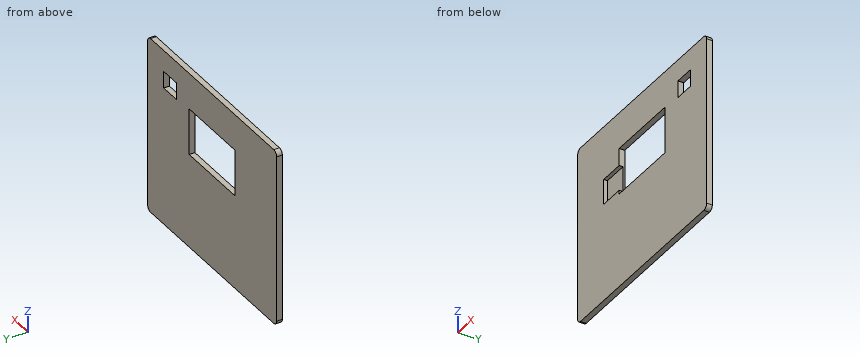
```python
from build123d import *

# Parameters (mm, degrees)
SKETCH_1_W               = 670
SKETCH_1_H               = 560
EXTRUDE_1_DEPTH          = 18
CUT_EXTRUDE_1_DEPTH      = 653.80088848
CUT_EXTRUDE_1_DEPTH_BACK = 653.80088848
SKETCH_2_W               = 65.5
SKETCH_2_H               = 53.5
CUT_EXTRUDE_2_DEPTH      = 653.80088848
CUT_EXTRUDE_2_DEPTH_BACK = 653.80088848
SKETCH_3_W               = 228
SKETCH_3_H               = 136
CUT_EXTRUDE_3_REACH      = 654.801
SKETCH_4_W               = 239
SKETCH_4_H               = 147
FILLET_1_R               = 15
SKETCH_8_W               = 80.472707968
SKETCH_8_H               = 80
CUT_EXTRUDE_4_DEPTH      = 12


with BuildPart() as part:
    # 草图1 → 凸台-拉伸1 (new body)
    with BuildSketch(Plane(origin=(0, 0, 0), x_dir=(1, 0, 0), z_dir=(0, 1, 0))):
        with Locations((0, 280)):
            Rectangle(SKETCH_1_W, SKETCH_1_H)
    extrude(amount=EXTRUDE_1_DEPTH)

    # 草图2 → 切除-拉伸1 (cut, two sides: drawn at the far end of the back side and taken through both)
    with BuildSketch(Plane(origin=(0, 18, 0), x_dir=(1, 0, 0), z_dir=(0, 1, 0)).offset(-CUT_EXTRUDE_1_DEPTH_BACK)):
        with Locations((218.822373939, 94.436899918)):
            Rectangle(SKETCH_2_W, SKETCH_2_H)
    extrude(amount=CUT_EXTRUDE_1_DEPTH + CUT_EXTRUDE_1_DEPTH_BACK, mode=Mode.SUBTRACT)

    # 草图3 → 切除-拉伸2 (cut, two sides: drawn at the far end of the back side and taken through both)
    with BuildSketch(Plane(origin=(0, 18, 0), x_dir=(1, 0, 0), z_dir=(0, 1, 0)).offset(-CUT_EXTRUDE_2_DEPTH_BACK)):
        with Locations((0, 188)):
            Rectangle(SKETCH_3_W, SKETCH_3_H)
    extrude(amount=CUT_EXTRUDE_2_DEPTH + CUT_EXTRUDE_2_DEPTH_BACK, mode=Mode.SUBTRACT)

    # 草图4 → 切除-拉伸3 (cut, up to next)
    with BuildSketch(Plane(origin=(0, 18, 0), x_dir=(1, 0, 0), z_dir=(0, 1, 0)), mode=Mode.PRIVATE) as cut_extrude_3_sk1:
        with Locations((0, 188)):
            Rectangle(SKETCH_4_W, SKETCH_4_H)
    cut_extrude_3_tool1 = extrude(cut_extrude_3_sk1.sketch, amount=-CUT_EXTRUDE_3_REACH, mode=Mode.PRIVATE) & part.part
    add(cut_extrude_3_tool1.solids().sort_by_distance((0, 18, -188))[0], mode=Mode.SUBTRACT)

    # 圆角1
    fillet_1_edges = [part.edges().sort_by_distance(p)[0] for p in [
        (-335, 9, -560),
        (335, 9, -560),
        (335, 9, 0),
        (-335, 9, 0),
    ]]
    fillet(fillet_1_edges, radius=FILLET_1_R)

    # 草图8 → 切除-拉伸4 (cut)
    with BuildSketch(Plane.XZ):
        with Locations((-159.736353984, -209.541384695)):
            Rectangle(SKETCH_8_W, SKETCH_8_H)
    extrude(amount=-CUT_EXTRUDE_4_DEPTH, mode=Mode.SUBTRACT)


solid = part.part
```
Verification items for the finished model (mm, model axes). Coordinates: 2 decimals unless noted, no trailing zeros. Write each loop counter-clockwise with the first axis right and the second up, starting at its lowest first coordinate (ties: lowest second). Pieces come first, ordered by that corner, then holes. Notation, with made-up numbers: M -14.75,-29 L 23.25,-29 A17 ccw 23.25,-16 Z; hole C -28,17 d11. An arc over 180 degrees is marked long. Answer as a JSON object with one key per item and string values. Group by question number.
(1) Gauge pin test, flat end, axial feed: pin 1 (12 mm diameter, centred on x = 117.5, z = -291, fed in from -Y). Record the tip position at first contact, or that the pin passes through.
(2) Cross-section at B-B, the plane z = -162. Record the cut outline in (x, y).
(3) Material ranges on line 1 (Z direction, x = 64, y = 6.25); line 2 (X direction, y = 12.25, z = -189); line 3 (X direction, y = 3.75, z = -174), recorded low to high.
(4) Cross-section at A-A, the plane x = 240. Record the cut outline in (y, z), and give its area (3 significant figures).
(5) Cross-section at C-C, the plane y = 4.5. Record the cut outline in (x, z).
Reply:
{
 "1": {"pin 1": "y = 0"},
 "2": {"outline": "M -335,0 L -119.5,0 L -119.5,18 L -335,18 Z; M 119.5,0 L 335,0 L 335,18 L 119.5,18 Z"},
 "3": {"line 1": "-560 to -261.5, -114.5 to 0", "line 2": "-335 to -119.5, 119.5 to 335", "line 3": "-335 to -199.97, 119.5 to 335"},
 "4": {"outline": "M 0,-560 L 18,-560 L 18,-121.19 L 0,-121.19 Z; M 0,-67.69 L 18,-67.69 L 18,0 L 0,0 Z", "area": "9,120 mm²"},
 "5": {"outline": "M -335,-545 A15 ccw -320,-560 L 320,-560 A15 ccw 335,-545 L 335,-15 A15 ccw 320,0 L -320,0 A15 ccw -335,-15 Z; hole M -199.97,-249.54 L -119.5,-249.54 L -119.5,-261.5 L 119.5,-261.5 L 119.5,-114.5 L -119.5,-114.5 L -119.5,-169.54 L -199.97,-169.54 Z; hole M 186.07,-121.19 L 251.57,-121.19 L 251.57,-67.69 L 186.07,-67.69 Z"}
}
